Model file for the job. Use its own axes, mm. Round coordinates to 2 decimals unless told otherwise and drop trailing zeros. Loops run counter-clockwise (first coordinate to the right, second up) from the corner with the lowest first, then second, coordinate; pieces in that order, holes last. Notation, with made-up numbers: (-12.5, 17) -> (25.5, 17) arc R23 cw to (25.5, 49) -> close; hole circle Ø9 at (65, 88). An arc over 180 degrees is marked (long way). Use a Markdown table: item, result.
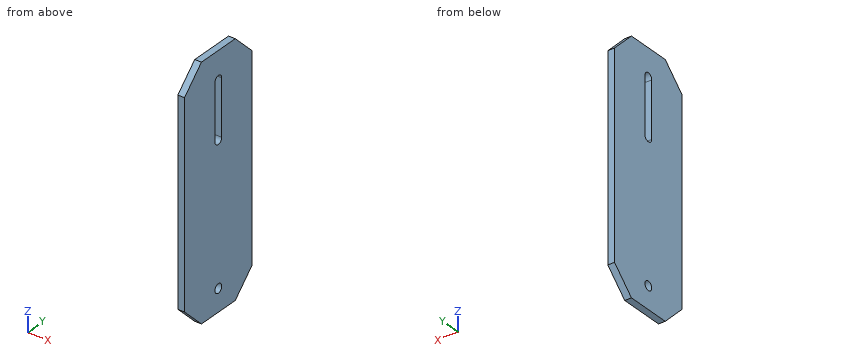
from build123d import *

# Parameters (mm, degrees)
SALIENTE_EXTRUIR1_DEPTH = 3
CROQUIS3_R              = 2
CORTAR_EXTRUIR1_DEPTH   = 9


with BuildPart() as part:
    # Croquis2 → Saliente-Extruir1 (new body)
    with BuildSketch(Plane(origin=(0, 0, 0), x_dir=(0, 0, -1), z_dir=(1, 0, 0))):
        Polygon((0, 0), (90, 0), (100, 10), (100, 30), (90, 40), (0, 40), (-10, 30), (-10, 10), align=None)
    extrude(amount=SALIENTE_EXTRUIR1_DEPTH)

    # Croquis3 → Cortar-Extruir1 (cut)
    with BuildSketch(Plane(origin=(3, 0, 0), x_dir=(0, 0, -1), z_dir=(1, 0, 0))):
        with Locations((90, 20)):
            Circle(CROQUIS3_R)
        with BuildLine():
            Line((2.5, 22), (27.5, 22))
            ThreePointArc((27.5, 22), (29.5, 20), (27.5, 18))
            Line((27.5, 18), (2.5, 18))
            ThreePointArc((2.5, 18), (0.5, 20), (2.5, 22))
        make_face()
    extrude(amount=-CORTAR_EXTRUIR1_DEPTH, mode=Mode.SUBTRACT)


solid = part.part
Q1. Drill centre lines: L1, parallel to Y at x = 2.2, z = -90; L2, parallel to Y at x = 2.6, z = -91.5; L3, parallel to Y at x = 1.45, z = -95. Where is each one in solid material? Low to high. Write a range as from..to.
Results list:
| item | result |
|---|---|
| L1 | y = 0..18, 22..40 |
| L2 | y = 1.5..18.68, 21.32..38.5 |
| L3 | y = 5..35 |
Q2. Band-saw the part on C-C, the plane z = 3.5. Give the cut face in (x, y).
Results list:
| item | result |
|---|---|
| outline | (0, 3.5) -> (3, 3.5) -> (3, 36.5) -> (0, 36.5) -> close |
Q3. Band-saw the part on A-A, the plane y = 20. Give the cut face in (x, z), plus the area to 3 significant figures.
Results list:
| item | result |
|---|---|
| outline | (0, -100) -> (3, -100) -> (3, -92) -> (0, -92) -> close; (0, -88) -> (3, -88) -> (3, -29.5) -> (0, -29.5) -> close; (0, -0.5) -> (3, -0.5) -> (3, 10) -> (0, 10) -> close |
| area | 231 mm² |
Q4. Band-saw the part on B-B, the plane x = 0.95. Give the cut face in (y, z).
Results list:
| item | result |
|---|---|
| outline | (0, -90) -> (10, -100) -> (30, -100) -> (40, -90) -> (40, 0) -> (30, 10) -> (10, 10) -> (0, 0) -> close; hole circle Ø4 at (20, -90); hole (18, -27.5) arc R2 ccw to (22, -27.5) -> (22, -2.5) arc R2 ccw to (18, -2.5) -> close |
